Check sheet for the drawn part. Datum: minimum x, y, z corner. Units: mm. Give positions to 0.01 mm unless a question says otherwise; leave off trailing zeros. Write each loop counter-clockwise with the first axis right and the second up, starting at its lowest first coordinate (ties: lowest second). Pieces come first, ordered by that corner, then holes. Notation, with made-up numbers: M 16.25,-32.5 L 72.25,-32.5 A13 cw 72.25,-12.5 Z; hole C -24,50.5 d5. An arc over 180 degrees is marked long. Write item = value, one per line.
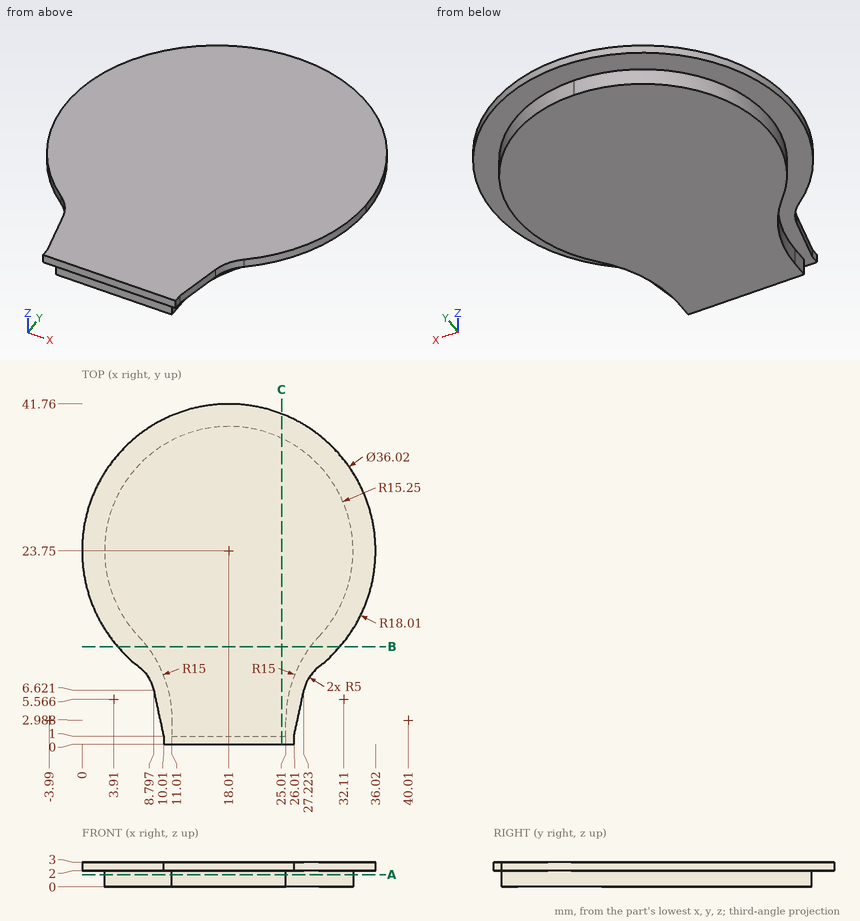
1) Depth check by flat-ended pin: P1, Ø1.1, axis at y = 0.5, z = 2.5, coming from the -X side; P2, Ø1, axis at x = 17, z = 2, coming from the +Y side; P3, Ø3, axis at x = 4, y = 37.5, coming from the -Z side; P4, Ø1, axis at x = 20.5, z = 1, coming from the -Y side. Enter the tip coordinate at first touch or a pass-through.
From the geometry:
P1 = 10
P2 = 41.75
P3 = through
P4 = 1
2) Material ranges on probe 1 along Z at (x, y) = (33, 29); probe 2 along X at (y, z) = (22, 1.9); probe 3 along X at (y, z) = (7, 2.5), recorded low to high. Write a range as from..to.
From the geometry:
probe_1 = 2..3
probe_2 = 2.86..33.16
probe_3 = 8.7..27.32
3) Cross-section at B-B on y = 12. Record the boundary of the cut face in (x, z).
From the geometry:
outline = M 4.36,2 L 8,2 L 8,0 L 28.02,0 L 28.02,2 L 31.66,2 L 31.66,3 L 4.36,3 Z
4) Cross-section at A-A on z = 1.5. Record the boundary of the cut face in (x, y).
From the geometry:
outline = M 6.92,13.28 A15 cw 11.01,2.99 L 11.01,1 L 25.01,1 L 25.01,2.99 A15 cw 29.1,13.28 A15.25 ccw long Z
5) Cross-section at C-C on x = 24.5. Record the boundary of the cut face in (y, z), plus the area to 3 significant figures.
From the geometry:
outline = M 0,2 L 1,2 L 1,0 L 37.55,0 L 37.55,2 L 40.55,2 L 40.55,3 L 0,3 Z
area = 114 mm^2
